Autodesk Inventor part; units mm, degrees
ref_plane "YZ Plane" through (0, 0, 0) normal (1, 0, 0) x (0, 1, 0)
ref_plane "XZ Plane" through (0, 0, 0) normal (0, 1, 0) x (-1, 0, 0)
ref_plane "XY Plane" through (0, 0, 0) normal (0, 0, 1) x (1, 0, 0)
sketch "스케치1" plane through (0, 0, 0) normal (0, 0, 1) x (1, 0, 0)
  circle A0 centre (0, 0) radius 5.5
  circle A1 centre (0, 0) radius 4.3
  dimension "d0" = 11
  dimension "d1" = 8.6
extrude "돌출1" add sketch "스케치1" along normal blind 13
sketch "스케치2" plane through (0, 0, 13) normal (0, 0, 1) x (1, 0, 0)
  circle A0 centre (0, 0) radius 4.3
  circle A1 centre (0, 0) radius 7.5
  dimension "d4" = 15
extrude "돌출2" add sketch "스케치2" along normal blind 3 contours A0 | A1
sketch "스케치3" plane through (0, 0, 0) normal (1, 0, 0) x (0, 1, 0)
  line L0 (7.4799, 10.5) -> (-8.5589, 10.5)
  line L1 (-8.5589, 10.5) -> (-8.5589, 12)
  line L2 (-8.5589, 12) -> (7.4799, 12)
  line L3 (7.4799, 12) -> (7.4799, 10.5)
  line L4 (7.5, 13) -> (-7.5, 13)
  point P0 (0, 0)
  dimension "d7" = 1.5
  dimension "d10" = 2.5
revolve "회전1" cut sketch "스케치3" angle 360 about axis through (0, 7.4799, 10.5) along (0, -1, 0)
properties part number "SAFRS-P-0060"
Work out the finished part from the listing and answer in its coordinate system (mm). A direction names the side the tool comes from. Round coordinates to 2 decimals unless told otherwise and drop trailing zeros. Write each loop counter-clockwise with the first axis right and the second up, starting at its lowest first coordinate (ties: lowest second). Pieces come first, ordered by that corner, then holes. Notation, with made-up numbers: (50, 61) -> (103, 61) arc R19 cw to (103, 79) -> close; hole circle Ø6 at (2, 80.5). An arc over 180 degrees is marked (long way). Write each question's results on one line, items separated by ' | '.
1) The part is cut by section B-B (z = 10.5). Write down the section's boundary in (x, y).
Findings:
outline: (-1.5, -5.29) -> (-1.5, -4.03) arc R4.3 cw to (-1.5, 4.03) -> (-1.5, 5.29) arc R5.5 ccw to start; (1.5, -5.29) arc R5.5 ccw to (1.5, 5.29) -> (1.5, 4.03) arc R4.3 cw to (1.5, -4.03) -> close
2) The part is cut by section D-D (x = 4). Write down the section's boundary in (y, z), and give its area (3 significant figures).
Findings:
outline: (-6.34, 13) -> (-3.77, 13) -> (-3.77, 0) -> (-1.58, 0) -> (-1.58, 13) -> (1.58, 13) -> (1.58, 0) -> (3.77, 0) -> (3.77, 13) -> (6.34, 13) -> (6.34, 16) -> (-6.34, 16) -> close | area: 95.2 mm²
3) For a pull along Z with two mould halves and no side action, classify faces 1 (the cylindrical face through (-7.493, -0.33, 14.479)), 2 (the flat face through (0, 0, 16)), 3 (the cylindrical face through (-0.575, 4.775, 11.886)) as +Z half, -Z half, draft (parallel to the pull), parting line (faces both ways), or undercut.
Findings:
face 1: draft | face 2: +Z half | face 3: undercut
4) Consider line 1 along Z through (x, y) = (0, 4.9); line 2 along Z through (x, y) = (-4, 5.75); line 3 along Y through (x, z) = (2.25, 6). Determine where each line is inside the solid, lowest interval first. Write a range as [from, to].
Findings:
line 1: z = [0, 9], [12, 16] | line 2: z = [13, 16] | line 3: y = [-5.02, -3.66], [3.66, 5.02]
5) Which of the six approach directions +Z, -Z, +X, -X, +Y, -Y give full straight-line access (tool end or side, diameter ignored) to faces 4 (the cylindrical face through (-1.464, -4.755, 10.175)), 5 (the cylindrical face through (1.984, 3.815, 6.409))?
Findings:
face 4: +Y, -Y | face 5: -Z
6) The part is cut by section C-C (y = 0). Write down the section's boundary in (x, z).
Findings:
outline: (-7.5, 13) -> (-5.5, 13) -> (-5.5, 0) -> (-4.3, 0) -> (-4.3, 13) -> (4.3, 13) -> (4.3, 0) -> (5.5, 0) -> (5.5, 13) -> (7.5, 13) -> (7.5, 16) -> (-7.5, 16) -> close
7) Flat-ended cylindrical pins translate along their axes: pin 1 (6 mm diameter, centred on x = -6, y = 2.5, fed in from -Z); pin 2 (5 mm diameter, centred on x = -4.5, z = 12, fed in from +Y); pin 3 (3 mm diameter, centred on y = 4, z = 9, fed in from -X); pin 4 (2.5 mm diameter, centred on x = 2, y = 1, fed in from -Z). Find the tip coordinate at first contact, or state that the pin passes through.
Findings:
pin 1: stops at z = 0 | pin 2: stops at y = 7.17 | pin 3: stops at x = -4.9 | pin 4: stops at z = 13
8) The part is cut by section A-A (x = 0). Write down the section's boundary in (y, z), and give its area (3 significant figures).
Findings:
outline: (-7.5, 13) -> (-5.5, 13) -> (-5.5, 12) -> (-4.3, 12) -> (-4.3, 13) -> (4.3, 13) -> (4.3, 12) -> (5.5, 12) -> (5.5, 13) -> (7.5, 13) -> (7.5, 16) -> (-7.5, 16) -> close; (-5.5, 0) -> (-4.3, 0) -> (-4.3, 9) -> (-5.5, 9) -> close; (4.3, 0) -> (5.5, 0) -> (5.5, 9) -> (4.3, 9) -> close | area: 69.0 mm²
